```python
from build123d import *

# Parameters (mm, degrees)
PLATE_SKETCH_W          = 76.2
PLATE_SKETCH_H          = 228.6
PLATE_EXTRUDE_DEPTH     = 6.35
F_1_4_CLEARANCE_HOLE2_D = 6.7564
F_6_CLEARANCE_HOLE1_D   = 3.7973
F_3_8_CLEARANCE_HOLE1_D = 10.0838


with BuildPart() as part:
    # Plate sketch → Plate extrude (new body)
    with BuildSketch(Plane(origin=(0, 0, 0), x_dir=(1, 0, 0), z_dir=(0, 1, 0))):
        Rectangle(PLATE_SKETCH_W, PLATE_SKETCH_H)
    extrude(amount=PLATE_EXTRUDE_DEPTH)

    # 1/4 Clearance Hole2 (through all)
    with Locations(Plane(origin=(0, 6.35, 0), x_dir=(1, 0, 0), z_dir=(0, 1, 0))):
        with Locations((-20.066, 79.375), (20.066, -12.7), (-20.066, -12.7), (20.066, 79.375)):
            Hole(F_1_4_CLEARANCE_HOLE2_D / 2)

    # #6 Clearance Hole1 (through all)
    with Locations(Plane(origin=(0, 6.35, 0), x_dir=(1, 0, 0), z_dir=(0, 1, 0))):
        with Locations((-31.75, -50.8), (-31.75, -109.5375), (31.75, -50.8), (31.75, -109.5375)):
            Hole(F_6_CLEARANCE_HOLE1_D / 2)

    # 3/8 Clearance Hole1 (through all)
    with Locations(Plane(origin=(0, 6.35, 0), x_dir=(1, 0, 0), z_dir=(0, 1, 0))):
        with Locations((-26.19375, 101.6), (26.19375, 101.6)):
            Hole(F_3_8_CLEARANCE_HOLE1_D / 2)


solid = part.part
```
Geometry: final body of the model. Coordinates: model frame, mm. Round coordinates to 2 decimals unless told otherwise and drop trailing zeros. Order: outer loops, then holes, each group sorted by start corner. A loop starts at its lowest first (then second) coordinate and runs counter-clockwise, first axis right, second up. Notation, with made-up numbers: M -27.5,-8 L 19.5,-8 A16 ccw 19.5,12 Z; hole C 41,-5.75 d10. An arc over 180 degrees is marked long. One line per item, written item: value.
(1) Cut plane C-C (z = 12.7). Return the cut outline in (x, y), and give its area (3 significant figures).
Result sheet:
outline: M -38.1,0 L -23.44,0 L -23.44,6.35 L -38.1,6.35 Z; M -16.69,0 L 16.69,0 L 16.69,6.35 L -16.69,6.35 Z; M 23.44,0 L 38.1,0 L 38.1,6.35 L 23.44,6.35 Z
area: 398 mm2
(2) Cut plane A-A (z = -101.6). Return the cut outline in (x, y).
Result sheet:
outline: M -38.1,0 L -31.24,0 L -31.24,6.35 L -38.1,6.35 Z; M -21.15,0 L 21.15,0 L 21.15,6.35 L -21.15,6.35 Z; M 31.24,0 L 38.1,0 L 38.1,6.35 L 31.24,6.35 Z
(3) Line query: probe 1 along X at (y, z) = (5, 50.8); probe 2 along Z at (x, y) = (-31.75, 4.75); probe 3 along X at (y, z) = (4.75, 12.7). Output: solid intervals per line, ascending. Write a range as [from, to].
Result sheet:
probe 1: [-38.1, -33.65], [-29.85, 29.85], [33.65, 38.1]
probe 2: [-114.3, 48.9], [52.7, 107.64], [111.44, 114.3]
probe 3: [-38.1, -23.44], [-16.69, 16.69], [23.44, 38.1]
(4) Cut plane B-B (y = 4). Give the number of separate pieces and of enclosed holes in the cut face, and give its area (3 significant figures).
Result sheet:
separate pieces: 1
enclosed holes: 10
area: 17,100 mm2
(5) Pull-direction query (X, two-part tool) for faces 1 (the flat face through (38.1, 3, 2)), 2 (the cylindrical face through (-33.504, 3.131, 51.527)), 3 (the flat face through (-38.1, 3, 2)), 4 (the flat face through (-1, 3, 114.3)); classes: pulls with the +X half, pulls with the -X half, needs draft (parallel to the pull), parting line crosses it, or undercut.
Result sheet:
face 1: pulls with the +X half
face 2: undercut
face 3: pulls with the -X half
face 4: needs draft
(6) Pin query (flat end, axial travel): P1, Ø6, axis at x = 20.066, z = -79.375, coming from the +Y side. Return the tip coordinate at first contact, or that it passes through.
Result sheet:
P1: through
